from build123d import *

# Parameters (mm, degrees)
PAD_DEPTH = 400


with BuildPart() as part:
    # Sketch → Pad (new body)
    with BuildSketch(Plane.XZ):
        Polygon((-7.5, 0), (7.5, 0), (7.5, 2.7), (5, 5.2), (5, 7.2), (7.5, 9.7), (7.5, 12.5), (5, 15), (-5, 15), (-7.5, 12.5), (-7.5, 9.7), (-5, 7.2), (-5, 5.2), (-7.5, 2.7), align=None)
    extrude(amount=PAD_DEPTH)


solid = part.part
Geometry check sheet. Reference: the model listing, model coordinates, mm. Round coordinates to 2 decimals unless told otherwise and drop trailing zeros. Write each loop counter-clockwise with the first axis right and the second up, starting at its lowest first coordinate (ties: lowest second). Pieces come first, ordered by that corner, then holes. Notation, with made-up numbers: (-34, 73) - (19, 73) arc R19 ccw to (19, 83) - close; hole circle Ø1 at (-22, 31). An arc over 180 degrees is marked (long way). One line per item, written item: value.
1. Cross-section at A-A on y = -220. Record the boundary of the cut face in (x, z).
The answers:
outline: (-7.5, 0) - (7.5, 0) - (7.5, 2.7) - (5, 5.2) - (5, 7.2) - (7.5, 9.7) - (7.5, 12.5) - (5, 15) - (-5, 15) - (-7.5, 12.5) - (-7.5, 9.7) - (-5, 7.2) - (-5, 5.2) - (-7.5, 2.7) - close
2. Scan lines: L1, parallel to Z at x = 6.75, y = -159; L2, parallel to Z at x = -6.5, y = -294; L3, parallel to X at y = -310.5, z = 6.5. Record each from-to range of solid material in increasing order.
The answers:
L1: z = 0 to 3.45, 8.95 to 13.25
L2: z = 0 to 3.7, 8.7 to 13.5
L3: x = -5 to 5
3. Depth check by flat-ended pin: pin 1 Ø8 at (x, y) = (-5.5, -202) entering from +Z; pin 2 Ø1 at (y, z) = (-177.5, 6) entering from -X; pin 3 Ø1.6 at (y, z) = (-295, 6.5) entering from +X. Enter the tip coordinate at first touch or a pass-through.
The answers:
pin 1: stops at z = 15
pin 2: stops at x = -5
pin 3: stops at x = 5.1
